Geometry: see drawing. Coordinates: mm, zero at the bounding-box minimum. Give positions to 0.01 mm unless a question says otherwise; leave off trailing zeros. Write each loop counter-clockwise with the first axis right and the second up, starting at its lowest first coordinate (ties: lowest second). Pieces come first, ordered by that corner, then holes. Notation, with made-up numbers: (80, 51) -> (104, 51) arc R22 ccw to (104, 61) -> close; hole circle Ø7 at (-8.75, 65). An arc over 180 degrees is marked (long way). Write item = value, one per line.
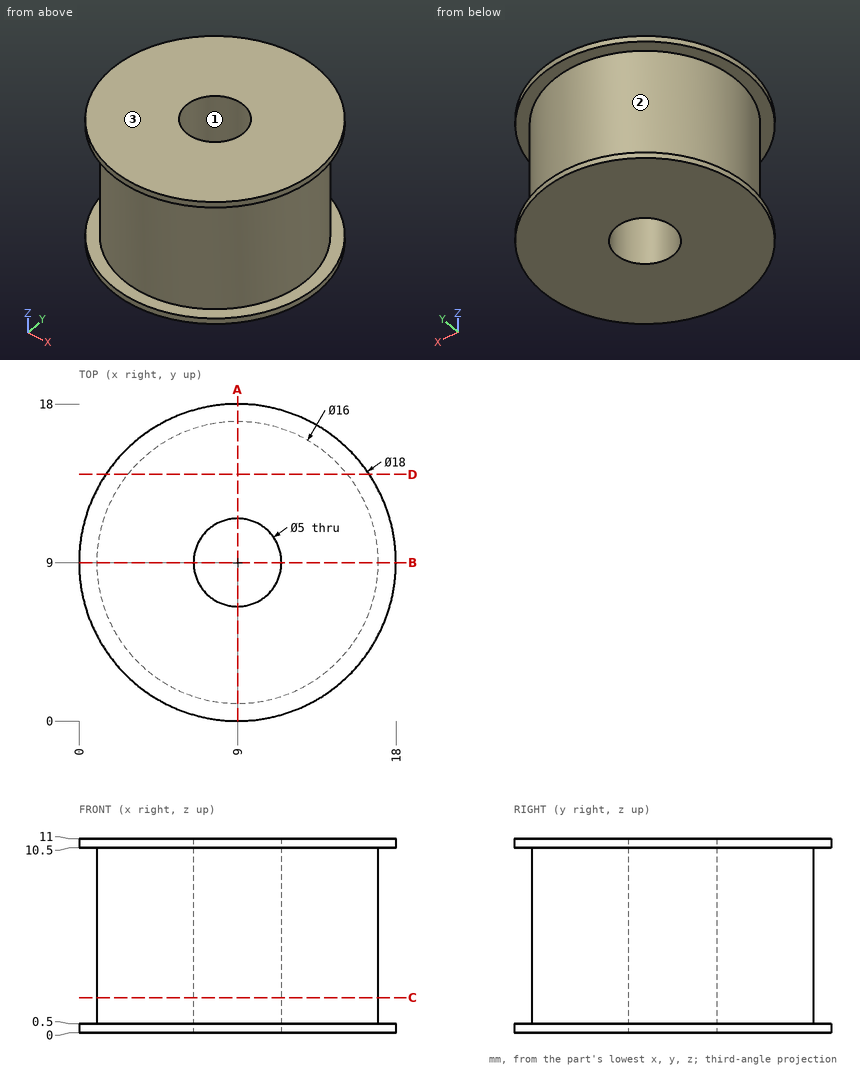
(1) First-contact query: pin 1 (1.5 mm diameter, centred on y = 10, z = 7.5, fed in from -X); pin 2 (4 mm diameter, centred on x = 7, y = 7, fed in from -Z); pin 3 (3 mm diameter, centred on y = 3.5, z = 8.5, fed in from -X); pin 4 (3 mm diameter, centred on y = 16, z = 5, fed in from -X). Flat tips, straight axial feed; report the tip coordinate or a pass-through.
Values follow:
pin_1 = 1
pin_2 = 0
pin_3 = 2.07
pin_4 = 3.19
(2) Section query C-C (z = 2). Return loops of the section in (x, y), plus the area to 3 significant figures.
Values follow:
outline = circle Ø16 at (9, 9); hole circle Ø5 at (9, 9)
area = 181 mm2
(3) Section query D-D (y = 14). Return loops of the section in (x, z) (3 decimals).
Values follow:
outline = (1.517, 0) -> (16.483, 0) -> (16.483, 0.5) -> (15.245, 0.5) -> (15.245, 10.5) -> (16.483, 10.5) -> (16.483, 11) -> (1.517, 11) -> (1.517, 10.5) -> (2.755, 10.5) -> (2.755, 0.5) -> (1.517, 0.5) -> close
(4) Pull-direction query (Z, two-part tool) for the marked faces 1, 2 and 3; classes: pulls with the +Z half, pulls with the -Z half, needs draft (parallel to the pull), parting line crosses it, or undercut.
Values follow:
face_1 = needs draft
face_2 = undercut
face_3 = pulls with the +Z half
(5) Material intervals for line 1 (Y direction, x = 9, z = 4.5); line 2 (Z direction, x = 7, y = 17); line 3 (Y direction, x = 6.75, z = 10), sorted ascending.
Values follow:
line_1 = 1 to 6.5, 11.5 to 17
line_2 = 0 to 0.5, 10.5 to 11
line_3 = 1.32 to 7.91, 10.09 to 16.68
(6) Section query A-A (x = 9). Return loops of the section in (y, z).
Values follow:
outline = (0, 0) -> (6.5, 0) -> (6.5, 11) -> (0, 11) -> (0, 10.5) -> (1, 10.5) -> (1, 0.5) -> (0, 0.5) -> close; (11.5, 0) -> (18, 0) -> (18, 0.5) -> (17, 0.5) -> (17, 10.5) -> (18, 10.5) -> (18, 11) -> (11.5, 11) -> close
